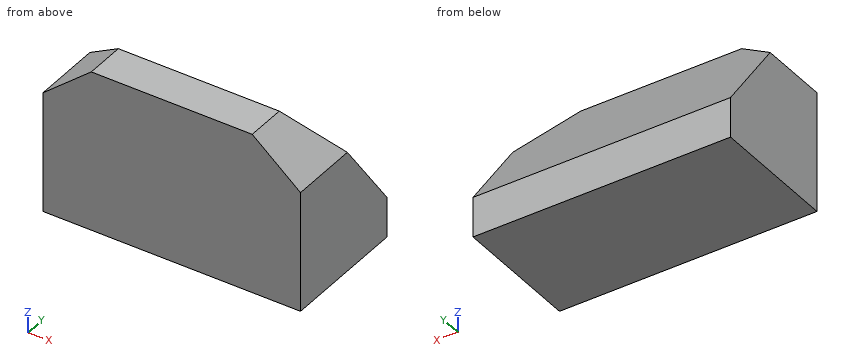
```python
from build123d import *

# Parameters (mm, degrees)
BOSS_EXTRUDE1_DEPTH = 101.6
CUT_EXTRUDE1_DEPTH  = 101.6
CUT_EXTRUDE2_DEPTH  = 101.6


with BuildPart() as part:
    # Sketch1 → Boss-Extrude1 (new body)
    with BuildSketch(Plane(origin=(0, 0, 0), x_dir=(0, 0, -1), z_dir=(1, 0, 0))):
        Polygon((0, 0), (63.5, 0), (63.5, 50.8), (47.625, 50.8), (0, 15.875), align=None)
    extrude(amount=-BOSS_EXTRUDE1_DEPTH)

    # Sketch3 → Cut-Extrude1 (cut)
    with BuildSketch(Plane.XZ):
        Polygon((0, 0), (-19.05, 0), (0, -15.875), align=None)
    extrude(amount=-CUT_EXTRUDE1_DEPTH, mode=Mode.SUBTRACT)

    # Sketch4 → Cut-Extrude2 (cut)
    with BuildSketch(Plane.XZ):
        Polygon((-101.6, 0), (-82.55, 0), (-101.6, -15.875), align=None)
    extrude(amount=-CUT_EXTRUDE2_DEPTH, mode=Mode.SUBTRACT)


solid = part.part
```
Read the model definition and answer for the solid it produces. Units are mm, in the model's axes. Coordinates: 2 decimals unless noted, no trailing zeros. Write each loop counter-clockwise with the first axis right and the second up, starting at its lowest first coordinate (ties: lowest second). Pieces come first, ordered by that corner, then holes. Notation, with made-up numbers: (-20.75, -12.75) -> (22.25, -12.75) arc R31 cw to (22.25, 23.25) -> close; hole circle Ø9 at (10.5, 17). An arc over 180 degrees is marked (long way). Answer as a JSON object with one key per item and string values.
Q1. The part is cut by section D-D on y = 19.5. Give the vertices of the cut face in (x, z) (3 decimals), then the cut area to 3 significant figures.
The answers:
{"outline": "(-101.6, -63.5) -> (0, -63.5) -> (0, -15.875) -> (-13.118, -4.943) -> (-88.482, -4.943) -> (-101.6, -15.875) -> close", "area": "5,810 mm2"}
Q2. Consider line 1 (Z direction, x = -28, y = 46); line 2 (Z direction, x = -33.5, y = 26.5); line 3 (Y direction, x = -44, z = -28.5) (3 decimals). Determine where each line is inside the solid, lowest interval first. Write a range as [from, to].
The answers:
{"line 1": "z = [-63.5, -41.08]", "line 2": "z = [-63.5, -14.49]", "line 3": "y = [0, 36.775]"}
Q3. The part is cut by section B-B on y = 5.5. Give the vertices of the cut face in (x, z) (3 decimals), then the cut area to 3 significant figures.
The answers:
{"outline": "(-101.6, -63.5) -> (0, -63.5) -> (0, -15.875) -> (-19.05, 0) -> (-82.55, 0) -> (-101.6, -15.875) -> close", "area": "6,150 mm2"}
Q4. The part is cut by section C-C on z = -3.5. Give the vertices of the cut face in (x, y).
The answers:
{"outline": "(-86.75, 0) -> (-14.85, 0) -> (-14.85, 18.44) -> (-86.75, 18.44) -> close"}
Q5. The part is cut by section A-A on x = -57. Give the vertices of the cut face in (y, z) (3 decimals), then the cut area to 3 significant figures.
The answers:
{"outline": "(0, -63.5) -> (50.8, -63.5) -> (50.8, -47.625) -> (15.875, 0) -> (0, 0) -> close", "area": "2,390 mm2"}
Q6. Flat-ended cylindrical pins translate along their axes: pin 1 Ø6 at (x, y) = (-83, 35) entering from +Z; pin 2 Ø1.5 at (x, z) = (-36.5, -9.5) entering from +Y; pin 3 Ø4 at (x, z) = (-68, -19) entering from +Y (3 decimals). Find the tip coordinate at first contact, or state that the pin passes through.
The answers:
{"pin 1": "stops at z = -21.99", "pin 2": "stops at y = 23.39", "pin 3": "stops at y = 31.275"}
